from build123d import *

# Parameters (mm, degrees)
SKETCH1_R           = 1.75
BOSS_EXTRUDE1_DEPTH = 57.5
BOSS_EXTRUDE2_DEPTH = 8.4
SKETCH3_W           = 5.3
SKETCH3_H           = 35
CUT_EXTRUDE1_DEPTH  = 5.4
CUT_EXTRUDE2_DEPTH  = 3.1
SKETCH5_W           = 18.2
SKETCH5_H           = 8.4
SKETCH5_W_2         = 8.4
SKETCH5_H_2         = 8.937392322
SKETCH5_W_3         = 9.875614017
SKETCH5_H_3         = 12.4
CUT_EXTRUDE3_DEPTH  = 18
LPATTERN1_COUNT     = 2
LPATTERN1_PITCH     = 27


with BuildPart() as part:
    # Sketch1 → Boss-Extrude1 (new body)
    with BuildSketch(Plane.XY):
        with BuildLine():
            Line((-52.8, -2.1), (-4.2, -2.1))
            Line((-4.2, -2.1), (-4.2, 0))
            ThreePointArc((-4.2, 0), (0, 4.2), (4.2, 0))
            Line((4.2, 0), (4.2, -2.1))
            Line((4.2, -2.1), (33.3, -2.1))
            Line((33.3, -2.1), (33.3, 0))
            ThreePointArc((33.3, 0), (34.530151519, 2.969848481), (37.5, 4.2))
            Line((37.5, 4.2), (41.5, 4.2))
            Line((41.5, 4.2), (41.5, -4.2))
            Line((41.5, -4.2), (-57, -4.2))
            ThreePointArc((-57, -4.2), (-60.217386661, -2.699707961), (-61.136192563, 0.729322346))
            Line((-61.136192563, 0.729322346), (-59.818910528, 8.2))
            Line((-59.818910528, 8.2), (-57, 8.2))
            Line((-57, 8.2), (-57, 4.2))
            Line((-57, 4.2), (-52.8, 4.2))
            Line((-52.8, 4.2), (-52.8, -2.1))
        make_face()
        Circle(SKETCH1_R, mode=Mode.SUBTRACT)
        with Locations((-57, 0)):
            Circle(SKETCH1_R, mode=Mode.SUBTRACT)
        with Locations((37.5, 0)):
            Circle(SKETCH1_R, mode=Mode.SUBTRACT)
    extrude(amount=BOSS_EXTRUDE1_DEPTH)

    # Sketch2 → Boss-Extrude2 (add)
    with BuildSketch(Plane(origin=(0, 4.2, 0), x_dir=(1, 0, 0), z_dir=(0, 1, 0))):
        Polygon((41.5, -57.5), (51.5, -57.5), (51.5, -17.5), (41.5, 0), align=None)
    extrude(amount=-BOSS_EXTRUDE2_DEPTH)

    # Sketch3 → Cut-Extrude1 (cut)
    with BuildSketch(Plane(origin=(0, 4.2, 0), x_dir=(1, 0, 0), z_dir=(0, 1, 0))):
        with Locations((47.35, -36.75)):
            Rectangle(SKETCH3_W, SKETCH3_H)
    extrude(amount=-CUT_EXTRUDE1_DEPTH, mode=Mode.SUBTRACT)

    # Sketch4 → Cut-Extrude2 (cut, through all)
    with BuildSketch(Plane(origin=(0, -2.1, 0), x_dir=(1, 0, 0), z_dir=(0, 1, 0))):
        with BuildLine():
            Line((-44.921320344, -49.378679656), (-42.8, -47.257359313))
            Line((-42.8, -47.257359313), (-40.678679656, -49.378679656))
            ThreePointArc((-40.678679656, -49.378679656), (-42.8, -54.5), (-44.921320344, -49.378679656))
        make_face()
    cut_extrude2 = extrude(amount=-CUT_EXTRUDE2_DEPTH, mode=Mode.SUBTRACT)

    # Sketch5 → Cut-Extrude3 (cut)
    with BuildSketch(Plane(origin=(0, 0, 0), x_dir=(-1, 0, 0), z_dir=(0, 0, -1))):
        with Locations((-42.4, 0)):
            Rectangle(SKETCH5_W, SKETCH5_H)
        with Locations((0, 0.268696161)):
            Rectangle(SKETCH5_W_2, SKETCH5_H_2)
        with Locations((57.737807008, 2)):
            Rectangle(SKETCH5_W_3, SKETCH5_H_3)
    extrude(amount=-CUT_EXTRUDE3_DEPTH, mode=Mode.SUBTRACT)

    # LPattern1: Cut-Extrude2 ×2
    with Locations(*[(i * LPATTERN1_PITCH, 0, 0) for i in range(1, LPATTERN1_COUNT)]):
        add(cut_extrude2, mode=Mode.SUBTRACT)


solid = part.part
Geometry: final body of the model. Coordinates: model frame, mm. A direction names the side the tool comes from. Give positions to 0.01 mm unless a question says otherwise; leave off trailing zeros. Loops run counter-clockwise (first coordinate to the right, second up) from the corner with the lowest first, then second, coordinate; pieces in that order, holes last. Notation, with made-up numbers: M 30,-35.5 L 52,-35.5 A21 ccw 52,-16.5 Z; hole C 40,-24 d10. An arc over 180 degrees is marked long. Put each result on its own line as item: value. Start each with the question number.
1) Ray query, line 1 along X through (y, z) = (-3.1, 51.5); line 2 along Z through (x, y) = (-42.8, -3.5); line 3 along X through (y, z) = (-1.25, 51). Return the intervals inside material, ascending.
2) Cut plane B-B (x = 0). Output: boundary loops of the cut face in (y, z).
3) Cut plane D-D (z = 39). Output: boundary loops of the cut face in (x, y), then the cut area to 3 significant figures.
4) Contact query for flat-ended pins moving along their axis: pin 1 (2.5 mm diameter, centred on y = -3.5, z = 10.5, fed in from +X); pin 2 (10 mm diameter, centred on x = 18, z = 17.5, fed in from +Y); pin 3 (1.3 mm diameter, centred on x = -54, z = 34.5, fed in from +Y). Output: stop coordinate, or through.
5) Cut plane A-A (z = 51.5). Give the number of separate pieces and of enclosed holes in the cut face, then the cut area to 3 significant figures.
6) Access query for faces 1 (the cylindrical face through (34.5, 2.94, 37.47)), 2 (the flat face through (50, 2, 37)), 3 (the cylindrical face through (-15.7, -3.1, 54.5)), 4 (the flat face through (4.2, -3, 9)), 5 (the flat face through (43, 0, 18)). Directions: +Z, -Z, +X, -X, +Y, -Y. A direction counts if a zero-diameter tool reaches every point of the face in a straight line with its end or side. Return the directions, or none.
7) Pull-direction query (Z, two-part tool) for faces 6 (the flat face through (19, -3, 0)), 7 (the flat face through (-16.876, -3.135, 48.333)), 8 (the flat face through (-41.754, -3.135, 48.303)), 9 (the flat face through (-52.8, -3, 9)); classes: pulls with the +Z half, pulls with the -Z half, needs draft (parallel to the pull), parting line crosses it, or undercut.
8) Cut plane C-C (z = 8.5). Output: boundary loops of the cut face in (x, y), then the cut area to 3 significant figures.
Verdict:
1. line 1: -59.83 to -45.8, -39.8 to -18.8, -12.8 to 51.5
1. line 2: 0 to 47.26, 54.5 to 57.5
1. line 3: -61.01 to -58.22, -55.78 to -52.8, -4.2 to -1.22, 1.22 to 4.2, 33.3 to 36.28, 38.72 to 51.5
2. outline: M -4.2,18 L -1.75,18 L -1.75,57.5 L -4.2,57.5 Z; M 1.75,18 L 4.2,18 L 4.2,57.5 L 1.75,57.5 Z
3. outline: M -61.14,0.73 A4.2 ccw -57,-4.2 L 51.5,-4.2 L 51.5,4.2 L 50,4.2 L 50,-1.2 L 44.7,-1.2 L 44.7,4.2 L 37.5,4.2 A4.2 ccw 33.3,0 L 33.3,-2.1 L 4.2,-2.1 L 4.2,0 A4.2 ccw -4.2,0 L -4.2,-2.1 L -52.8,-2.1 L -52.8,4.2 L -57,4.2 L -57,8.2 L -59.82,8.2 Z; hole C -57,0 d3.5; hole C 0,0 d3.5; hole C 37.5,0 d3.5
3. area: 396 mm2
4. pin 1: x = 33.3
4. pin 2: y = -2.1
4. pin 3: y = 4.2
5. separate pieces: 3
5. enclosed holes: 3
5. area: 371 mm2
6. face 1: +Z, -Z, +Y
6. face 2: +Y
6. face 3: +Y, -Y
6. face 4: -Z, +Y, -Y
6. face 5: -Z, +X, +Y, -Y
7. face 6: pulls with the -Z half
7. face 7: undercut
7. face 8: undercut
7. face 9: needs draft
8. outline: M -52.8,-4.2 L -4.2,-4.2 L -4.2,-2.1 L -52.8,-2.1 Z; M 4.2,-4.2 L 33.3,-4.2 L 33.3,-2.1 L 4.2,-2.1 Z
8. area: 163 mm2
